The drawing under review shows one solid part. Ordinate dimensions are in mm from its lowest x, y, z. A direction names the side the tool comes from. Coordinates: 2 decimals unless noted, no trailing zeros. Write each loop counter-clockwise with the first axis right and the second up, starting at its lowest first coordinate (ties: lowest second). Pieces come first, ordered by that corner, then holes.
Q1. Add section A-A, the plane x = 23. Give the boundary of the cut face in (y, z) (3 decimals).
Q2. Machinability: for the marked faces 1 and 2, which of the approach directions +Z, -Z, +X, -X, +Y, -Y give a long, thin tool a straight path to every point of the face, cutting with its end or side? Answer none if there is none.
Q3. To check wall thickness, follow probe 1 along X at (y, z) = (2.05, 140); probe 2 along Z at (x, y) = (23, 8.3); probe 3 along Y at (x, z) = (19.5, 154) (3 decimals). State the ranges of each line that lie inside material, in increasing order.
Q4. Clearance check with flat-ended pins moving along their axes: pin 1 Ø3 at (x, y) = (50, 60) entering from +Z; pin 2 Ø11 at (x, z) = (23, 140) entering from +Y; pin 3 Ø0.5 at (x, y) = (73.5, 5) entering from +Z. State where each tip first meets the part, or that it passes through.
Q5. Add section B-B, the plane z = 140. Give the number of separate pieces and of enclosed holes in the cut face, plus the area to 3 significant figures.
Q6. Add section D-D, the plane y = 45.5. Give the boundary of the cut face in (x, z), plus the area to 3 significant figures.
Q7. Add section C-C, the plane x = 9. Give the boundary of the cut face in (y, z) (3 decimals), plus the area to 3 significant figures.
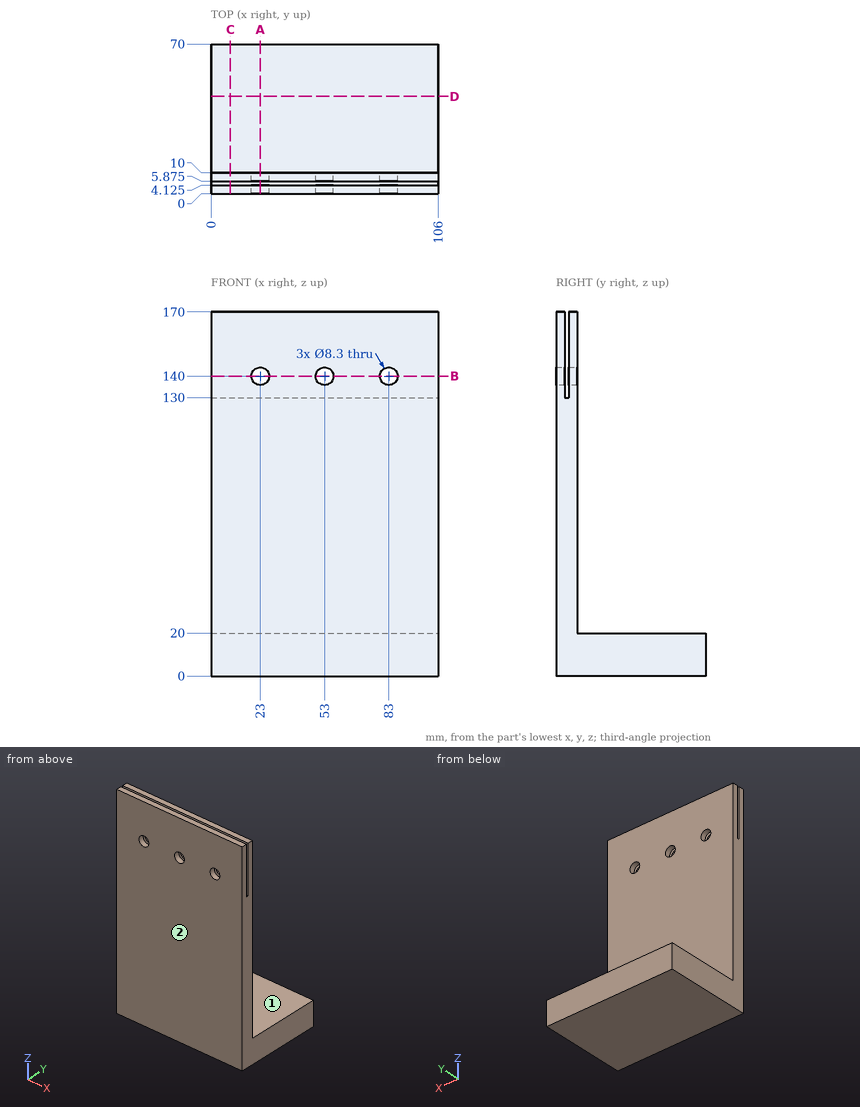
Here are the results:
1. outline: (0, 0) - (70, 0) - (70, 20) - (10, 20) - (10, 135.85) - (5.875, 135.85) - (5.875, 130) - (4.125, 130) - (4.125, 135.85) - (0, 135.85) - close; (0, 144.15) - (4.125, 144.15) - (4.125, 170) - (0, 170) - close; (5.875, 144.15) - (10, 144.15) - (10, 170) - (5.875, 170) - close
2. face 1: +Z, +X, -X, +Y
2. face 2: +Z, -Z, +X, -X, -Y
3. probe 1: x = 0 to 18.85, 27.15 to 48.85, 57.15 to 78.85, 87.15 to 106
3. probe 2: z = 0 to 135.85, 144.15 to 170
3. probe 3: y = 0 to 4.125, 5.875 to 10
4. pin 1: stops at z = 20
4. pin 2: stops at y = 10
4. pin 3: stops at z = 130
5. separate pieces: 8
5. enclosed holes: 0
5. area: 669 mm2
6. outline: (0, 0) - (106, 0) - (106, 20) - (0, 20) - close
6. area: 2,120 mm2
7. outline: (0, 0) - (70, 0) - (70, 20) - (10, 20) - (10, 170) - (5.875, 170) - (5.875, 130) - (4.125, 130) - (4.125, 170) - (0, 170) - close
7. area: 2,830 mm2
